Autodesk Inventor part; units mm, degrees
ref_plane "YZ Plane" through (0, 0, 0) normal (1, 0, 0) x (0, 1, 0)
ref_plane "XZ Plane" through (0, 0, 0) normal (0, 1, 0) x (-1, 0, 0)
ref_plane "XY Plane" through (0, 0, 0) normal (0, 0, 1) x (1, 0, 0)
sketch "Sketch1" plane through (0, 0, 0) normal (0, 1, 0) x (-1, 0, 0)
  line L0 (-100, -260) -> (100, -260)
  line L1 (100, -260) -> (100, 260)
  line L2 (100, 260) -> (-100, 260)
  line L3 (-100, 260) -> (-100, -260)
  line L4 (-100, -260) -> (100, 260) construction
  line L5 (100, -260) -> (-100, 260) construction
  point P0 (0, 0)
  dimension "d0" = 200
  dimension "d1" = 520
extrude "Extrusion1" add sketch "Sketch1" along normal blind 10
fillet "Fillet1" radius 25 4 edges at (-100, 5, -260) (-100, 5, 260) (100, 5, 260) (100, 5, -260)
sketch "Sketch2" plane through (0, 10, 0) normal (0, 1, 0) x (1, 0, 0)
  line L0 (100, -235) -> (100, 235)
  line L1 (-75, -260) -> (75, -260)
  point P0 (0, 0)
  point P1 (85, -245)
  dimension "d5" = 15
  dimension "d6" = 15
hole "Hole1" at (85, 10, 245) direction (0, -1, 0) diameter 6.647 end through all
pattern_linear "Rectangular Pattern1" count 2 spacing 170 along (-1, 0, 0) count 2 spacing 490 along (0, 0, -1) of "Hole1"
sketch "Sketch3" plane through (0, 10, 0) normal (0, 1, 0) x (1, 0, 0)
  line L0 (-75, -260) -> (75, -260)
  line L1 (-100, 235) -> (-100, -235)
  point P0 (0, 0)
  point P1 (-10, -245)
  point P2 (55, -245)
  dimension "d20" = 15
  dimension "d21" = 90
  dimension "d22" = 65
  dimension "d23" = 15
hole "Hole2" at (-10, 10, 245) at (55, 10, 245) direction (0, -1, 0) diameter 6.647 end through all
mirror "Mirror1" about plane through (0, 0, 0) normal (0, 0, 1) of "Hole2"
sketch "Sketch4" plane through (0, 10, 0) normal (0, 1, 0) x (1, 0, 0)
  line L0 (75, 260) -> (-75, 260)
  line L1 (100, -235) -> (100, 235)
  point P0 (0, 0)
  point P1 (-45, 30)
  point P2 (85, 30)
  dimension "d31" = 230
  dimension "d32" = 145
  dimension "d33" = 230
  dimension "d34" = 15
hole "Hole3" at (-45, 10, -30) at (85, 10, -30) direction (0, -1, 0) diameter 6.647 end through all
sketch "Sketch8" plane through (0, 10, 0) normal (0, 1, 0) x (1, 0, 0)
  line L0 (-100, 235) -> (-100, -235)
  line L1 (-100, -125) -> (-75, -125)
  line L2 (-75, -125) -> (-75, -195)
  line L3 (-75, -195) -> (-100, -195)
  line L4 (-100, -195) -> (-100, -125)
  line L5 (-75, -260) -> (75, -260)
  point P0 (0, 0)
  dimension "d72" = 25
  dimension "d73" = 70
  dimension "d74" = 65
extrude "Extrusion2" cut sketch "Sketch8" against normal blind 10
fillet "Fillet2" radius 10 4 edges at (-100, 5, 125) (-75, 5, 125) (-100, 5, 195) (-75, 5, 195)
sketch "Sketch9" plane through (0, 10, 0) normal (0, 1, 0) x (1, 0, 0)
  line L0 (-55, 50) -> (-85, 50)
  line L1 (-85, 50) -> (-85, -50)
  line L2 (-85, -50) -> (-55, -50)
  line L3 (-55, -50) -> (-55, 50)
  line L4 (-100, 235) -> (-100, -115)
  line L5 (75, 260) -> (-75, 260)
  point P0 (0, 0)
  dimension "d78" = 30
  dimension "d79" = 100
  dimension "d80" = 15
  dimension "d81" = 210
extrude "Extrusion3" cut sketch "Sketch9" against normal blind 10
fillet "Fillet3" radius 15 4 edges at (-55, 5, -50) (-55, 5, 50) (-85, 5, 50) (-85, 5, -50)
sketch "Sketch10" plane through (0, 10, 0) normal (0, 1, 0) x (1, 0, 0)
  line L0 (-30, 180) -> (-60, 180)
  line L1 (-60, 180) -> (-60, 110)
  line L2 (-60, 110) -> (-30, 110)
  line L3 (-30, 110) -> (-30, 180)
  line L4 (-100, 235) -> (-100, -115)
  line L5 (75, 260) -> (-75, 260)
  point P0 (0, 0)
  dimension "d85" = 30
  dimension "d86" = 70
  dimension "d87" = 40
  dimension "d88" = 80
extrude "Extrusion4" cut sketch "Sketch10" against normal blind 10
fillet "Fillet4" radius 15 4 edges at (-60, 5, -110) (-60, 5, -180) (-30, 5, -180) (-30, 5, -110)
sketch "Sketch11" plane through (0, 10, 0) normal (0, 1, 0) x (1, 0, 0)
  line L0 (-100, 235) -> (-100, -115)
  line L1 (-100, -205) -> (-100, -235)
  line L2 (75, 260) -> (-75, 260)
  line L3 (-75, -260) -> (75, -260)
  point P0 (0, 0)
  point P1 (-50, 220)
  point P2 (-50, 70)
  point P3 (-50, -80)
  point P4 (-50, -155)
  point P5 (-50, -230)
  dimension "d92" = 50
  dimension "d93" = 50
  dimension "d94" = 50
  dimension "d95" = 50
  dimension "d96" = 50
  dimension "d97" = 40
  dimension "d98" = 190
  dimension "d99" = 180
  dimension "d100" = 105
  dimension "d101" = 30
hole "Hole7" at (-50, 10, -220) at (-50, 10, -70) at (-50, 10, 80) at (-50, 10, 155) at (-50, 10, 230) direction (0, -1, 0) diameter 4.134 end through all
properties part number "Current_plate" material "Stainless Steel"
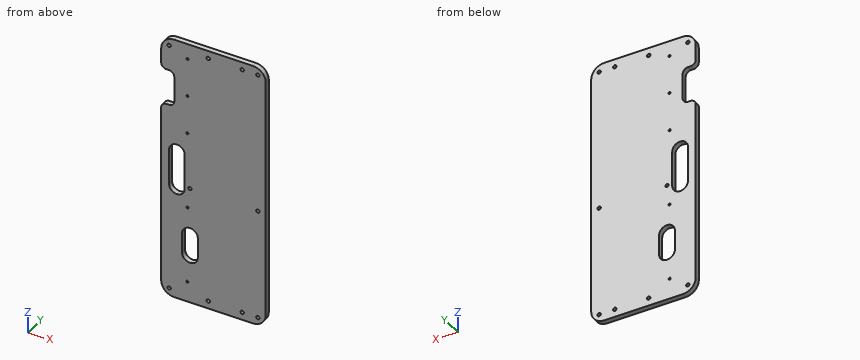
Here's how the part is built. I have some questions about the finished solid (model axes, mm). Give positions to 0.01 mm unless a question says otherwise; leave off trailing zeros. Use a Markdown table: item, result. Add a question column.
Item 1: I need wall thicknesses on line 1 (X direction, y = 1.75, z = -16.5); line 2 (X direction, y = 7, z = 245); line 3 (Z direction, x = -13, y = 5). Which ranges of each line are inside material? Lowest first, please.
Item 2: Will these pins go through, and if not, where does the flat tip stop? pin 1 (5 mm diameter, centred on x = 30, z = 184, fed in from -Y); pin 2 (2.5 mm diameter, centred on x = -50, z = -220, fed in from -Y); pin 3 (1 mm diameter, centred on x = -77, y = 6, fed in from +Z).
Item 3: Imagine slicing it at A-A on y = 4.25. Give the number of separate pieces and of enclosed holes in the cut face, plus the area to 3 significant figures.
Data:
| question | item | result |
|---|---|---|
| 1 | line 1 | x = -100 to -85, -55 to 100 |
| 1 | line 2 | x = -97.91 to -88.32, -81.68 to -13.32, -6.68 to 51.68, 58.32 to 81.68, 88.32 to 97.91 |
| 1 | line 3 | z = -260 to -246.43, -243.57 to 243.57, 246.43 to 260 |
| 2 | pin 1 | stops at y = 0 |
| 2 | pin 2 | passes through |
| 2 | pin 3 | stops at z = 259.95 |
| 3 | separate pieces | 1 |
| 3 | enclosed holes | 17 |
| 3 | area | 96,600 mm² |
